from build123d import *

# Parameters (mm, degrees)
ESQUISSE1_W             = 30
ESQUISSE1_H             = 30
BOSS_EXTRU_1_DEPTH      = 30
ENL_V_MAT_EXTRU_1_REACH = 47
ENL_V_MAT_EXTRU_2_REACH = 41.843
ESQUISSE4_R             = 3.25
ESQUISSE6_R             = 2.75
ENL_V_MAT_EXTRU_3_DEPTH = 10


with BuildPart() as part:
    # Esquisse1 → Boss.-Extru.1 (new body)
    with BuildSketch(Plane.XY):
        Rectangle(ESQUISSE1_W, ESQUISSE1_H)
    extrude(amount=BOSS_EXTRU_1_DEPTH)

    # Esquisse3 → Enlèv. mat.-Extru.1 (cut, up to next)
    with BuildSketch(Plane(origin=(0, 15, 0), x_dir=(1, 0, 0), z_dir=(0, 1, 0)), mode=Mode.PRIVATE) as enl_v_mat_extru_1_sk1:
        Polygon((-15, -20), (-5, -30), (-15, -30), align=None)
    enl_v_mat_extru_1_tool1 = extrude(enl_v_mat_extru_1_sk1.sketch, amount=-ENL_V_MAT_EXTRU_1_REACH, mode=Mode.PRIVATE) & part.part
    # Esquisse3 → Enlèv. mat.-Extru.1 (cut, up to next)
    with BuildSketch(Plane(origin=(0, 15, 0), x_dir=(1, 0, 0), z_dir=(0, 1, 0)), mode=Mode.PRIVATE) as enl_v_mat_extru_1_sk2:
        Polygon((-15, 0), (-15, -10), (-5, 0), align=None)
    enl_v_mat_extru_1_tool2 = extrude(enl_v_mat_extru_1_sk2.sketch, amount=-ENL_V_MAT_EXTRU_1_REACH, mode=Mode.PRIVATE) & part.part
    # Esquisse3 → Enlèv. mat.-Extru.1 (cut, up to next)
    with BuildSketch(Plane(origin=(0, 15, 0), x_dir=(1, 0, 0), z_dir=(0, 1, 0)), mode=Mode.PRIVATE) as enl_v_mat_extru_1_sk3:
        Polygon((15, 0), (5, 0), (15, -10), align=None)
    enl_v_mat_extru_1_tool3 = extrude(enl_v_mat_extru_1_sk3.sketch, amount=-ENL_V_MAT_EXTRU_1_REACH, mode=Mode.PRIVATE) & part.part
    # Esquisse3 → Enlèv. mat.-Extru.1 (cut, up to next)
    with BuildSketch(Plane(origin=(0, 15, 0), x_dir=(1, 0, 0), z_dir=(0, 1, 0)), mode=Mode.PRIVATE) as enl_v_mat_extru_1_sk4:
        Polygon((15, -30), (15, -20), (5, -30), align=None)
    enl_v_mat_extru_1_tool4 = extrude(enl_v_mat_extru_1_sk4.sketch, amount=-ENL_V_MAT_EXTRU_1_REACH, mode=Mode.PRIVATE) & part.part
    add(enl_v_mat_extru_1_tool1.solids().sort_by_distance((-11.666667, 15, 26.666667))[0], mode=Mode.SUBTRACT)
    add(enl_v_mat_extru_1_tool2.solids().sort_by_distance((-11.666667, 15, 3.333333))[0], mode=Mode.SUBTRACT)
    add(enl_v_mat_extru_1_tool3.solids().sort_by_distance((11.666667, 15, 3.333333))[0], mode=Mode.SUBTRACT)
    add(enl_v_mat_extru_1_tool4.solids().sort_by_distance((11.666667, 15, 26.666667))[0], mode=Mode.SUBTRACT)

    # Esquisse4 → Enlèv. mat.-Extru.2 (cut, up to next)
    with BuildSketch(Plane(origin=(-17.5, 0, 17.5), x_dir=(0.7071067811865489, 0, 0.7071067811865462), z_dir=(-0.7071067811865462, 0, 0.7071067811865489)), mode=Mode.PRIVATE) as enl_v_mat_extru_2_sk1:
        with Locations((10.605533906, -5)):
            Circle(ESQUISSE4_R)
    enl_v_mat_extru_2_tool1 = extrude(enl_v_mat_extru_2_sk1.sketch, amount=-ENL_V_MAT_EXTRU_2_REACH, mode=Mode.PRIVATE) & part.part
    add(enl_v_mat_extru_2_tool1.solids().sort_by_distance((-10.000755, -5, 24.999245))[0], mode=Mode.SUBTRACT)

    # Esquisse6 → Enlèv. mat.-Extru.3 (cut)
    with BuildSketch(Plane.XZ.offset(15)):
        with Locations(Location((0, 15, 0), (0, 0, 270))):
            Circle(ESQUISSE6_R)
    extrude(amount=-ENL_V_MAT_EXTRU_3_DEPTH, mode=Mode.SUBTRACT)


solid = part.part
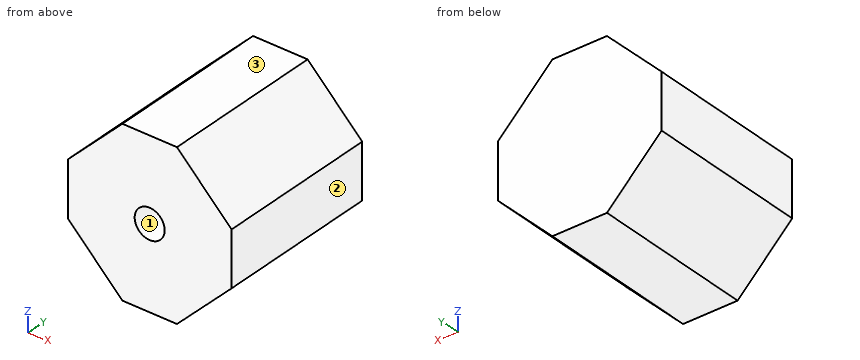
CAD build for the part. Positions are in the model's coordinates, mm. Face numbers are marked on the shaded views. Give positions to 0.01 mm unless a question says otherwise; leave off trailing zeros. Order: outer loops, then holes, each group sorted by start corner. A loop starts at its lowest first (then second) coordinate and runs counter-clockwise, first axis right, second up. Notation, with made-up numbers: (21.25, 63.5) -> (39.25, 63.5) arc R14 ccw to (39.25, 80.5) -> close; hole circle Ø5 at (48, -37.5). An arc over 180 degrees is marked (long way). Return JSON: item names as keys, results as strings.
Q1. Saw through at B-B (y = -0.5). Write the cut outline in (x, z), then the cut area to 3 significant figures.
Working result:
{"outline": "(-15, 10) -> (-5, 0) -> (5, 0) -> (15, 10) -> (15, 20) -> (5, 30) -> (-5, 30) -> (-15, 20) -> close", "area": "700 mm²"}
Q2. Mould opens along Z. For the marked faces 1, 2 and 3 say: pulls with the +Z half, pulls with the -Z half, needs draft (parallel to the pull), parting line crosses it, or undercut.
Working result:
{"face 1": "undercut", "face 2": "needs draft", "face 3": "pulls with the +Z half"}
Q3. Saw through at A-A (y = -11.5). Write the cut outline in (x, z), then the cut area to 3 significant figures.
Working result:
{"outline": "(-15, 10) -> (-5, 0) -> (5, 0) -> (15, 10) -> (15, 20) -> (5, 30) -> (-5, 30) -> (-15, 20) -> close; hole circle Ø5.5 at (0, 15)", "area": "676 mm²"}
Q4. Drill centre lines: line 1 (Z direction, x = 0, y = -10.5); line 2 (X direction, y = -12.5, z = 15); line 3 (Y direction, x = -7.5, z = 26). Where is each one in solid material? Low to high.
Working result:
{"line 1": "0 to 12.25, 17.75 to 30", "line 2": "-15 to -2.75, 2.75 to 15", "line 3": "-15 to -7.11, -2.89 to 15"}
Q5. Flat gauge pins, fed straight in: pin 1 (5 mm diameter, centred on y = -3, z = 23, fed in from -X); pin 2 (5 mm diameter, centred on x = -9, y = 3, fed in from +Z); pin 3 (1.5 mm diameter, centred on x = -8.5, y = -1.5, fed in from -Z). Where does each tip first touch, or does it go through?
Working result:
{"pin 1": "x = -14.5", "pin 2": "z = 28.5", "pin 3": "z = 2.75"}
